Can you work these out from the drawing? Everything is in mm from the part's minimum corner. A direction names the side the tool comes from. Round coordinates to 2 decimals unless told otherwise and drop trailing zeros. Loops run counter-clockwise (first coordinate to the right, second up) from the corner with the lowest first, then second, coordinate; pieces in that order, holes last. Notation, with made-up numbers: M 88,-37.5 L 141,-37.5 A5 ccw 141,-29.5 Z; hole C -24.75,-5.5 d3. An arc over 180 degrees is marked long. Return JSON: item names as keys, results as strings. Group by question number.
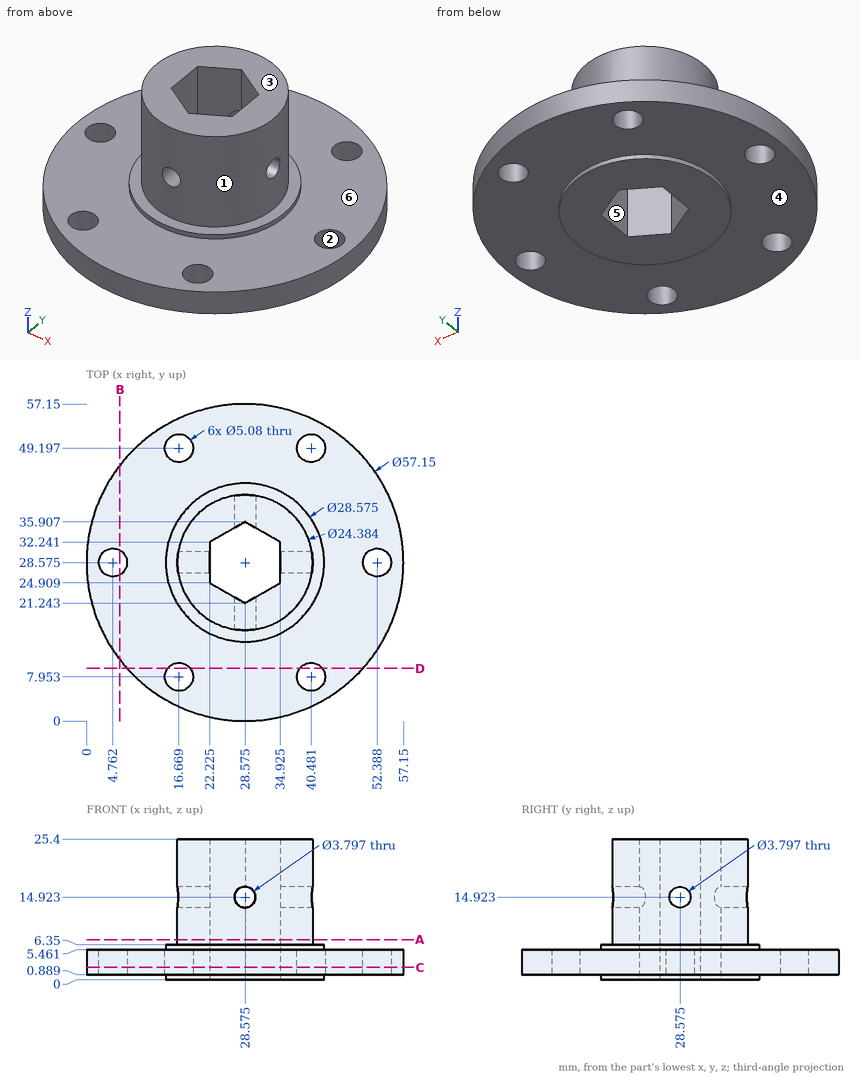
1. If we section it at C-C, the plane z = 2.25: Give the number of separate pieces and of enclosed holes in the cut face, then the cut area to 3 significant figures.
2. I need wall thicknesses on probe 1 along Z at (x, y) = (40, 4); probe 2 along Z at (x, y) = (30, 22) (1 decimal); probe 3 along Y at (x, z) = (24, 5.5) (1 decimal). Which ranges of each line are inside material? Lowest first, please.
3. We'd pull the mould along Y, two halves only. Please class the marked faces 1, 2 and 3: +Y half, -Y half, draft (parallel to the pull), parting line (faces both ways), or undercut.
4. If we section it at A-A, the plane z = 7.25: Please give me the cut outline in (x, y) (1 decimal).
5. I'm going to push flat-ended pins straight in: pin 1 Ø6 at (x, z) = (45, 12.5) entering from -Y; pin 2 Ø2 at (x, z) = (30.5, 22) entering from -Y; pin 3 Ø4.5 at (y, z) = (28.58, 14.92) entering from -X; pin 4 Ø6.5 at (x, y) = (52.39, 28.58) entering from -Z. Where does each tip first touch, or does it pass through?
6. If we section it at B-B, the plane x = 6: Please give me the cut outline in (y, z), then the cut area to 3 significant figures.
7. If we section it at D-D, the plane y = 9.5: Please give me the cut outline in (x, z) (1 decimal).
8. On a 3-axis mill with a long thin cutter (end or side, diameter ignored), from which of +Z, -Z, +X, -X, +Y, -Y can I reach the whole of each face in a straight line? I mean the marked faces 4, 5 and 6. Say none if no direction works.
Geometry results:
{
 "1": {"separate pieces": "1", "enclosed holes": "7", "area": "2,300 mm^2"},
 "2": {"probe 1": "0.89 to 5.46", "probe 2": "0 to 13.7, 16.2 to 25.4", "probe 3": "15 to 23.9, 33.3 to 42.1"},
 "3": {"face 1": "parting line", "face 2": "undercut", "face 3": "draft"},
 "4": {"outline": "C 28.6,28.6 d24.4; hole M 22.2,24.9 L 28.6,21.2 L 34.9,24.9 L 34.9,32.2 L 28.6,35.9 L 22.2,32.2 Z"},
 "5": {"pin 1": "through", "pin 2": "y = 16.42", "pin 3": "x = 16.38", "pin 4": "z = 0.89"},
 "6": {"outline": "M 11.06,0.89 L 26.36,0.89 L 26.36,5.46 L 11.06,5.46 Z; M 30.79,0.89 L 46.09,0.89 L 46.09,5.46 L 30.79,5.46 Z", "area": "140 mm^2"},
 "7": {"outline": "M 7.3,0.9 L 14.7,0.9 L 14.7,5.5 L 7.3,5.5 Z; M 18.7,0.9 L 38.5,0.9 L 38.5,5.5 L 18.7,5.5 Z; M 42.5,0.9 L 49.9,0.9 L 49.9,5.5 L 42.5,5.5 Z"},
 "8": {"face 4": "-Z", "face 5": "+Z, -Z", "face 6": "+Z"}
}
